The model under review builds one solid part; all positions refer to its coordinate system, in mm. A direction names the side the tool comes from. Coordinates: 2 decimals unless noted, no trailing zeros. Loops run counter-clockwise (first coordinate to the right, second up) from the corner with the lowest first, then second, coordinate; pieces in that order, holes last. Notation, with made-up numbers: (7.25, -25.5) - (32.25, -25.5) arc R8 cw to (32.25, -21.5) - close; hole circle Ø9 at (51.25, 69). An arc over 180 degrees is marked (long way). One line per item, written item: value. Start each with the question number.
1. To check wall thickness, follow line 1 (Z direction, x = 0, y = 2.2); line 2 (X direction, y = 3, z = -47.5); line 3 (X direction, y = 3.25, z = -12). State the ranges of each line that lie inside material, in increasing order.
2. We need section C-C, the plane y = 6.5. Give the boundary of the cut face in (x, z).
3. We need section A-A, the plane z = -5. Give the boundary of the cut face in (x, y).
4. For faces 1 (the face through (19.9, 4.1, -3.6)), 2 (the face through (-10, 0, -29)), list the 3-axis set-ups (+Z, -Z, +X, -X, +Y, -Y) from which the entire face can be reached by the end or side of a thin tool; tool diameter is ignored.
5. We need section B-B, the plane x = 0. Give the boundary of the cut face in (y, z).
6. We need section D-D, the plane z = -47.5. Give the boundary of the cut face in (x, y).
7. Insertion check: P1, Ø4, axis at x = -18.5, z = -5, coming from the -Y side; P2, Ø5.5, axis at x = 0, z = -12, coming from the +Y side. Each pin has a flat end and moves straight along its axis. Give the tip position at first contact, or say it passes through.
8. Mouldability with a two-part tool opening along Z and no side actions: class faces 3 (the face through (-17.1, 4.1, -3.6)), 4 (the face through (15.253, 5.824, -5.143)), 5 (the face through (0, 4, -73)), 6 (the face through (0, 4, 0)) as +Z half, -Z half, draft (parallel to the pull), parting line (faces both ways), or undercut.
from build123d import *

# Parameters (mm, degrees)
SKETCH1_W                                           = 45
SKETCH1_H                                           = 73
SKETCH1_R                                           = 20.25
BOSS_EXTRUDE1_DEPTH                                 = 7.5
CHAMFER1_SIZE                                       = 4
CBORE_FOR_M3_HEX_SOCKET_HEAD_CAP_SCREW1_D           = 3.4
CBORE_FOR_M3_HEX_SOCKET_HEAD_CAP_SCREW1_DEPTH       = 7.5
CBORE_FOR_M3_HEX_SOCKET_HEAD_CAP_SCREW1_CBORE_D     = 6.5
CBORE_FOR_M3_HEX_SOCKET_HEAD_CAP_SCREW1_CBORE_DEPTH = 3.4


with BuildPart() as part:
    # Sketch1 → Boss-Extrude1 (new body)
    with BuildSketch(Plane(origin=(0, 0, 0), x_dir=(1, 0, 0), z_dir=(0, 1, 0))):
        with Locations((0, 36.5)):
            Rectangle(SKETCH1_W, SKETCH1_H)
        with Locations((0, 47.5)):
            Circle(SKETCH1_R, mode=Mode.SUBTRACT)
    extrude(amount=BOSS_EXTRUDE1_DEPTH)

    # Chamfer1
    chamfer1_edges = [part.edges().sort_by_distance(p)[0] for p in [
        (-22.5, 3.75, -73),
        (22.5, 3.75, -73),
    ]]
    chamfer(chamfer1_edges, length=CHAMFER1_SIZE)

    # CBORE for M3 Hex Socket Head Cap Screw1
    with Locations(Plane(origin=(0, 7.5, 0), x_dir=(1, 0, 0), z_dir=(0, 1, 0))):
        with Locations((-18.5, 5), (0, 12), (18.5, 5)):
            CounterBoreHole(CBORE_FOR_M3_HEX_SOCKET_HEAD_CAP_SCREW1_D / 2, CBORE_FOR_M3_HEX_SOCKET_HEAD_CAP_SCREW1_CBORE_D / 2, CBORE_FOR_M3_HEX_SOCKET_HEAD_CAP_SCREW1_CBORE_DEPTH, depth=CBORE_FOR_M3_HEX_SOCKET_HEAD_CAP_SCREW1_DEPTH)


solid = part.part
Findings below:
1. line 1: -73 to -67.75, -27.25 to -13.7, -10.3 to 0
1. line 2: -22.5 to -20.25, 20.25 to 22.5
1. line 3: -22.5 to -1.7, 1.7 to 22.5
2. outline: (-22.5, -69) - (-18.5, -73) - (18.5, -73) - (22.5, -69) - (22.5, 0) - (-22.5, 0) - close; hole circle Ø6.5 at (-18.5, -5); hole circle Ø40.5 at (0, -47.5); hole circle Ø6.5 at (0, -12); hole circle Ø6.5 at (18.5, -5)
3. outline: (-22.5, 0) - (-20.2, 0) - (-20.2, 4.1) - (-21.75, 4.1) - (-21.75, 7.5) - (-22.5, 7.5) - close; (-16.8, 0) - (16.8, 0) - (16.8, 4.1) - (15.25, 4.1) - (15.25, 7.5) - (-15.25, 7.5) - (-15.25, 4.1) - (-16.8, 4.1) - close; (20.2, 0) - (22.5, 0) - (22.5, 7.5) - (21.75, 7.5) - (21.75, 4.1) - (20.2, 4.1) - close
4. face 1: +Y
4. face 2: +Z, -Z, +X, -X, -Y
5. outline: (0, -73) - (7.5, -73) - (7.5, -67.75) - (0, -67.75) - close; (0, -27.25) - (7.5, -27.25) - (7.5, -15.25) - (4.1, -15.25) - (4.1, -13.7) - (0, -13.7) - close; (0, -10.3) - (4.1, -10.3) - (4.1, -8.75) - (7.5, -8.75) - (7.5, 0) - (0, 0) - close
6. outline: (-22.5, 0) - (-20.25, 0) - (-20.25, 7.5) - (-22.5, 7.5) - close; (20.25, 0) - (22.5, 0) - (22.5, 7.5) - (20.25, 7.5) - close
7. P1: y = 0
7. P2: y = 4.1
8. face 3: undercut
8. face 4: undercut
8. face 5: -Z half
8. face 6: +Z half
